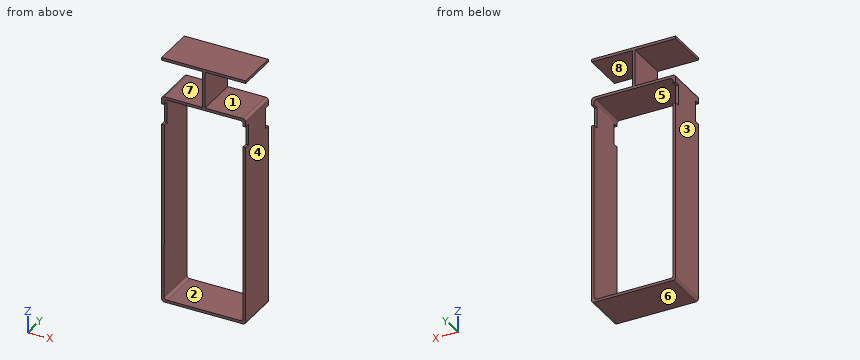
from build123d import *

# Parameters (mm, degrees)
F1_DEPTH = 50.8
F2_R     = 3.175
F3_W     = 19.05
F3_H     = 25.4
F3_W_2   = 6.35
F4_DEPTH = 127


with BuildPart() as f1:
    # F0 (on Front) → F1 (new body)
    with BuildSketch(Plane.XZ):
        Polygon((-7.708922, 210.136639), (-56.921422, 210.136639), (-56.921422, -43.863361), (44.678578, -43.863361), (44.678578, 210.136639), (-4.533922, 210.136639), (-4.533922, 254.586639), (44.678578, 254.586639), (44.678578, 257.761639), (-56.921422, 257.761639), (-56.921422, 254.586639), (-7.708922, 254.586639), align=None)
        Polygon((-53.746422, -40.688361), (-53.502657, 206.961519), (41.503578, 206.961519), (41.503578, -40.688361), align=None, mode=Mode.SUBTRACT)
    extrude(amount=F1_DEPTH)

    # F2
    f2_edges = [f1.edges().sort_by_distance(p)[0] for p in [
        (-56.921422, -25.4, 210.136639),
        (-53.502657, -25.4, 206.961519),
        (44.678578, -25.4, 210.136639),
        (41.503578, -25.4, 206.961519),
        (44.678578, -25.4, -43.863361),
        (41.503578, -25.4, -40.688361),
        (-56.921422, -25.4, -43.863361),
        (-53.746422, -25.4, -40.688361),
    ]]
    fillet(f2_edges, radius=F2_R)

    # F3 (on face) → F4 (cut)
    with BuildSketch(Plane.YZ.offset(44.678578)):
        with Locations((-60.325, 187.911639)):
            Rectangle(F3_W, F3_H)
        with Locations((-47.625, 187.911639)):
            Rectangle(F3_W_2, F3_H)
        with Locations((-3.175, 187.911639)):
            Rectangle(F3_W_2, F3_H)
    extrude(amount=-F4_DEPTH, mode=Mode.SUBTRACT)


solid = f1.part
Model file for the job. Use its own axes, mm. Face numbers are marked on the shaded views. A direction names the side the tool comes from. Round coordinates to 2 decimals unless told otherwise and drop trailing zeros. Order: outer loops, then holes, each group sorted by start corner. A loop starts at its lowest first (then second) coordinate and runs counter-clockwise, first axis right, second up. Notation, with made-up numbers: M 10,65 L 67,65 A17 ccw 67,69 Z; hole C -36,71 d1. An arc over 180 degrees is marked long. Write each question's results on one line, items separated by ' | '. Start each with the question number.
(1) Saw through at A-A, the plane x = -47. Give the cut face in (y, z), then the cut area to 3 significant figures.
(2) Which spindle directions (+Z, -Z, +X, -X, +Y, -Y) get a long thin tool onto all of the face, cutting with end or side? Do the marked faces 5, 6, 7 and 8. Say none if no direction does.
(3) Saw through at D-D, the plane z = 145.5. Give the cut face in (x, y), then the cut area to 3 significant figures.
(4) Two-plate mould, pull along X, no slides. Class the marked faces 1, 2, 3 and 4: pulls with the +X half, pulls with the -X half, needs draft (parallel to the pull), parting line crosses it, or undercut.
(5) Saw through at B-B, the plane z = -18. Give the cut face in (x, y).
(6) Probe probe 1 along Z at (x, y) = (-18.5, -22); probe 2 along X at (y, z) = (-15.5, 200.5); probe 3 along Z at (x, y) = (-6.5, -23.5). List the from-to ranges inside material, lowest first. Write a range as from..to.
(7) Saw through at C-C, the plane y = -35.5. Give the cut face in (x, z) (3 decimals), then the cut area to 3 significant figures.
(8) Drop flat-ended pins along their axis: pin 1 (1.7 mm diameter, centred on x = -55.5, y = -46.5, fed in from -Z); pin 2 (2.5 mm diameter, centred on x = -54.5, y = -4, fed in from -Z); pin 3 (22 mm diameter, centred on y = -31.5, z = 232, fed in from -X). Give the stop position or say it passes through.
Established:
1) outline: M -50.8,-43.86 L 0,-43.86 L 0,-40.69 L -50.8,-40.69 Z; M -50.8,206.96 L 0,206.96 L 0,210.14 L -50.8,210.14 Z; M -50.8,254.59 L 0,254.59 L 0,257.76 L -50.8,257.76 Z | area: 484 mm^2
2) face 5: +Y, -Y | face 6: -Z, +X, -X, +Y, -Y | face 7: -X, +Y, -Y | face 8: +X, +Y, -Y
3) outline: M -56.92,-50.8 L -53.56,-50.8 L -53.56,0 L -56.92,0 Z; M 41.5,-50.8 L 44.68,-50.8 L 44.68,0 L 41.5,0 Z | area: 332 mm^2
4) face 1: needs draft | face 2: undercut | face 3: pulls with the -X half | face 4: pulls with the +X half
5) outline: M -56.92,-50.8 L -53.72,-50.8 L -53.72,0 L -56.92,0 Z; M 41.5,-50.8 L 44.68,-50.8 L 44.68,0 L 41.5,0 Z
6) probe 1: z = -43.86..-40.69, 206.96..210.14, 254.59..257.76 | probe 2: x = -56.92..-53.51, 41.5..44.68 | probe 3: z = -43.86..-40.69, 206.96..257.76
7) outline: M -56.921,-40.688 A3.175 ccw -53.746,-43.863 L 41.504,-43.863 A3.175 ccw 44.679,-40.688 L 44.679,206.962 A3.175 ccw 41.504,210.137 L -4.534,210.137 L -4.534,254.587 L 44.679,254.587 L 44.679,257.762 L -56.921,257.762 L -56.921,254.587 L -7.709,254.587 L -7.709,210.137 L -53.746,210.137 A3.175 ccw -56.921,206.962 Z; hole M -53.743,-37.51 A3.175 ccw -50.568,-40.688 L 38.329,-40.688 A3.175 ccw 41.504,-37.513 L 41.504,203.787 A3.175 ccw 38.329,206.962 L -50.331,206.962 A3.175 ccw -53.506,203.79 Z | area: 2,710 mm^2
8) pin 1: stops at z = -43.73 | pin 2: stops at z = -43.86 | pin 3: stops at x = -7.71
